```python
from build123d import *

# Parameters (mm, degrees)
EXTRUDE_1_DEPTH = 6
M3X0_5_1_D      = 2.5
M3X0_5_1_DEPTH  = 4
M3X0_5_1_TIP    = 0.751075774
SKETCH_5_R      = 1.5
EXTRUDE_2_DEPTH = 5


with BuildPart() as part:
    # 草圖1 → 填料-伸長1 (new body)
    with BuildSketch(Plane.XY):
        Polygon((2.63, 0), (1.315, 2.277646812), (-1.315, 2.277646812), (-2.63, 0), (-1.315, -2.277646812), (1.315, -2.277646812), align=None)
    extrude(amount=EXTRUDE_1_DEPTH)

    # M3x0.5 螺紋孔1
    with Locations(Plane(origin=(0, 0, 0), x_dir=(-1, 0, 0), z_dir=(0, 0, -1))):
        with Locations((0, 0)):
            Hole(M3X0_5_1_D / 2, depth=M3X0_5_1_DEPTH)
            with Locations((0, 0, -(M3X0_5_1_DEPTH + M3X0_5_1_TIP / 2))):  # 118° drill point
                Cone(0, M3X0_5_1_D / 2, M3X0_5_1_TIP, mode=Mode.SUBTRACT)

    # 草圖5 → 填料-伸長2 (add)
    with BuildSketch(Plane.XY.offset(6)):
        Circle(SKETCH_5_R)
    extrude(amount=EXTRUDE_2_DEPTH)


solid = part.part
```
Can you work these out from the model? Positions are in its coordinate system, mm. A direction names the side the tool comes from. Coordinates: 2 decimals unless noted, no trailing zeros. Order: outer loops, then holes, each group sorted by start corner. A loop starts at its lowest first (then second) coordinate and runs counter-clockwise, first axis right, second up. Notation, with made-up numbers: (23, 63) - (68, 63) arc R31 ccw to (68, 88) - close; hole circle Ø2 at (-4.75, -0.5). An arc over 180 degrees is marked (long way). Answer in a Markdown table with one row per item.
1. For pin 1 (1.5 mm diameter, centred on y = -0.5, z = 3, fed in from +X), with a flat end and sliding along its axis, tell me the tip position at first contact or that it passes through.
Reply:
| item | result |
|---|---|
| pin 1 | stops at x = 2.63 |
2. For faces 4 (the cylindrical face through (-1.5, 0.07, 8.46)), 5 (the conical face through (0.05, -0.21, 4.62)), which set-ups out of +Z, -Z, +X, -X, +Y, -Y let a thin tool reach every point of the face, with its end or its side?
Reply:
| item | result |
|---|---|
| face 4 | +Z |
| face 5 | -Z |
3. If we mould it in two halves opening along Y, with no side actions, what happens to faces 1 (the flat face through (0, 2, 6)), 2 (the cylindrical face through (-0.27, -1.22, 2.03)), 3 (the flat face through (1.963, -1.155, 2.958))? For each: pulls with the +Y half, pulls with the -Y half, needs draft (parallel to the pull), parting line crosses it, or undercut.
Reply:
| item | result |
|---|---|
| face 1 | needs draft |
| face 2 | undercut |
| face 3 | pulls with the -Y half |
4. Suppose I cut it at A-A (z = 0.5). Please give me the cut outline in (x, y) (3 decimals).
Reply:
| item | result |
|---|---|
| outline | (-2.63, 0) - (-1.315, -2.278) - (1.315, -2.278) - (2.63, 0) - (1.315, 2.278) - (-1.315, 2.278) - close; hole circle Ø2.5 at (0, 0) |
5. If I drill on line 1 along Y through (x, z) = (0, 1.8); line 2 along X through (y, z) = (0.05, 2.5); line 3 along Z through (x, y) = (1.15, 1.45), over which ranges is the centre line in solid material (lowest first)?
Reply:
| item | result |
|---|---|
| line 1 | y = -2.28 to -1.25, 1.25 to 2.28 |
| line 2 | x = -2.6 to -1.25, 1.25 to 2.6 |
| line 3 | z = 0 to 6 |
6. Suppose I cut it at B-B (z = 10). Please give me the cut outline in (x, y).
Reply:
| item | result |
|---|---|
| outline | circle Ø3 at (0, 0) |
